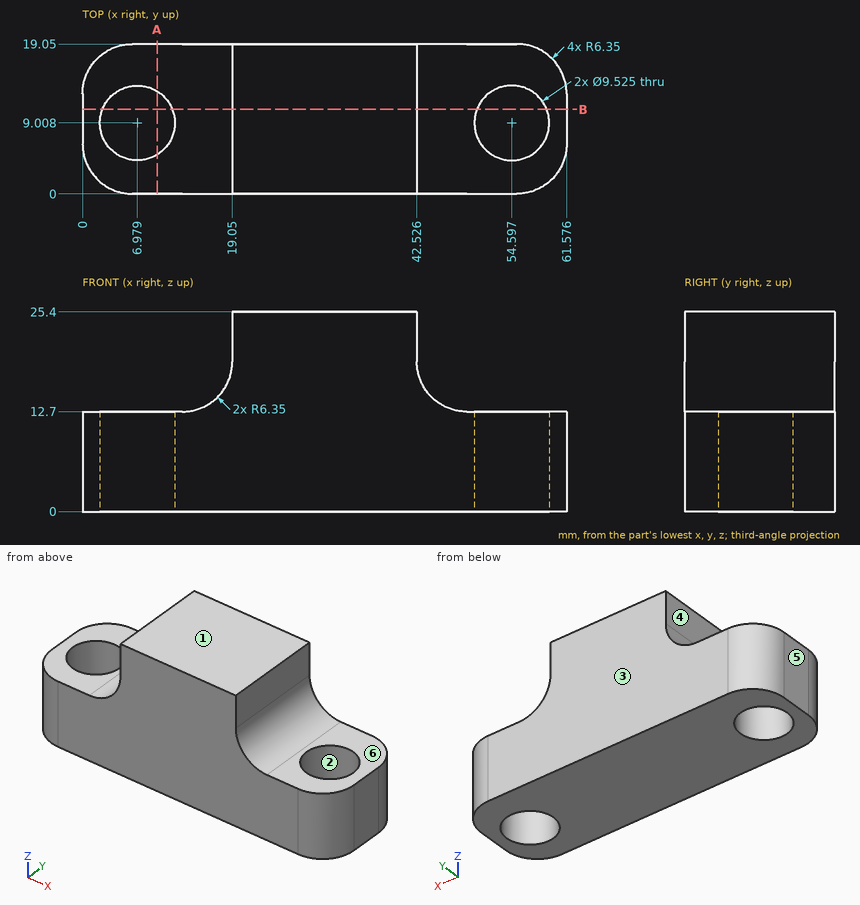
Job drawing, mm, ordinate dimensions from the low corner. One solid piece. A direction names the side the tool comes from. Give positions to 0.01 mm unless a question says otherwise; leave off trailing zeros. Write each loop counter-clockwise with the first axis right and the second up, starting at its lowest first coordinate (ties: lowest second). Pieces come first, ordered by that corner, then holes. Notation, with made-up numbers: M 73.5,-28.5 L 99.5,-28.5 A36 cw 99.5,10.5 Z; hole C 16.25,73 d4. An arc over 180 degrees is marked long. Put each result on its own line as item: value. Start each with the question number.
(1) Probe L1, parallel to X at y = 8.25, z = 12.25 (1 decimal); L2, parallel to X at y = 10.75, z = 3.75 (1 decimal); L3, parallel to X at y = 6, z = 22. List the from-to ranges inside material, lowest first.
(2) Which spindle directions (+Z, -Z, +X, -X, +Y, -Y) get a long thin tool onto all of the face, cutting with end or side? Do the marked faces 4, 5 and 6. Say none if no direction does.
(3) Mould opens along Y. For the marked faces 1, 2 and 3 say: +Y half, -Y half, draft (parallel to the pull), parting line (faces both ways), or undercut.
(4) Band-saw the part on A-A, the plane x = 9.5. Write the cut outline in (y, z).
(5) Flat gauge pins, fed straight in: pin 1 Ø5 at (y, z) = (8.5, 21) entering from -X; pin 2 Ø6.5 at (x, y) = (6.5, 11.5) entering from +Z; pin 3 Ø6 at (x, z) = (47.5, 13) entering from -Y; pin 4 Ø1 at (y, z) = (14.5, 18) entering from +X. Where does each tip first touch, or does it go through?
(6) Band-saw the part on B-B, the plane y = 10.75. Give the number of separate pieces and of enclosed holes in the cut face, and give its area (3 significant figures).
Response values:
1. L1: x = 0 to 2.3, 11.7 to 49.9, 59.3 to 61.6
1. L2: x = 0 to 2.5, 11.4 to 50.2, 59 to 61.6
1. L3: x = 19.05 to 42.53
2. face 4: +Z, -X, +Y, -Y
2. face 5: +Z, -Z, -X, +Y, -Y
2. face 6: +Z, +X, +Y, -Y
3. face 1: draft
3. face 2: undercut
3. face 3: +Y half
4. outline: M 0,0 L 4.97,0 L 4.97,12.7 L 0,12.7 Z; M 13.05,0 L 19.05,0 L 19.05,12.7 L 13.05,12.7 Z
5. pin 1: stops at x = 19.03
5. pin 2: stops at z = 12.7
5. pin 3: stops at y = 0
5. pin 4: stops at x = 42.72
6. separate pieces: 3
6. enclosed holes: 0
6. area: 872 mm2
